The listing builds one solid part. Answer for the finished solid, in the listing's coordinates (mm). Face numbers are marked on the shaded views. A direction names the side the tool comes from. Coordinates: 2 decimals unless noted, no trailing zeros. Order: outer loops, then holes, each group sorted by start corner. A loop starts at its lowest first (then second) coordinate and runs counter-clockwise, first axis right, second up. Notation, with made-up numbers: (89.25, -25) -> (138.25, -25) arc R32 cw to (138.25, 2) -> close; hole circle Ø2 at (43, 5.5). An arc over 180 degrees is marked (long way). Write item = value, one per line.
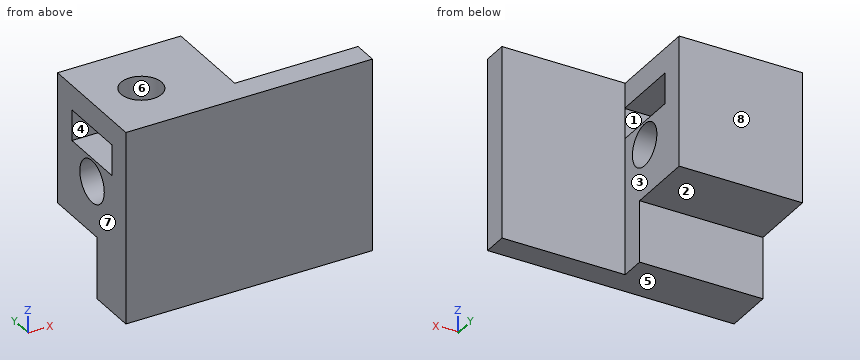
from build123d import *

# Parameters (mm, degrees)
RESSALTO_EXTRUS_O1_DEPTH             = 52.5
ESBO_O3_W                            = 10
ESBO_O3_H                            = 4
RESSALTO_EXTRUS_O2_DEPTH             = 5
ESBO_O4_R                            = 1.7
ESBO_O4_W                            = 2.5
ESBO_O4_H                            = 5.6
RESSALTO_EXTRUS_O3_DEPTH             = 10
ESBO_O5_R                            = 1.65
CORTE_EXTRUS_O1_DEPTH                = 6
RESSALTO_EXTRUS_O4_REACH             = 12.6
ESBO_O6_W                            = 10
ESBO_O6_H                            = 2
RESSALTO_EXTRUS_O4_DIRECTION_2_REACH = 117.6
ESBO_O7_W                            = 20
ESBO_O7_H                            = 110.6
CORTE_EXTRUS_O2_DEPTH                = 6.5
CORTE_EXTRUS_O2_DEPTH_BACK           = 5


with BuildPart() as part:
    # Esboço1 → Ressalto-extrusão1 (new body, symmetric)
    with BuildSketch(Plane.XY):
        Polygon((0, 0), (0, 2), (5, 2), (5, 4), (10, 4), (10, 2), (20, 2), (20, 0), align=None)
    extrude(amount=RESSALTO_EXTRUS_O1_DEPTH, both=True)

    # Esboço3 → Ressalto-extrusão2 (add)
    with BuildSketch(Plane.XY.offset(52.5)):
        with Locations((5, 2)):
            Rectangle(ESBO_O3_W, ESBO_O3_H)
    extrude(amount=-RESSALTO_EXTRUS_O2_DEPTH)

    # Esboço4 → Ressalto-extrusão3 (add, through all)
    with BuildSketch(Plane(origin=(10, 0, 0), x_dir=(0, 0, -1), z_dir=(1, 0, 0))):
        Polygon((-52.5, 9.5), (-63.1, 9.5), (-63.1, 0), (-52.5, 0), (-52.5, 3.742943079), align=None)
        with Locations((-56.7, 4.7)):
            Circle(ESBO_O4_R, mode=Mode.SUBTRACT)
        with Locations((-59.85, 4.7)):
            Rectangle(ESBO_O4_W, ESBO_O4_H, mode=Mode.SUBTRACT)
    ressalto_extrus_o3 = extrude(amount=-RESSALTO_EXTRUS_O3_DEPTH)

    # Esboço5 → Corte-extrusão1 (cut)
    with BuildSketch(Plane.XY.offset(63.1)):
        with Locations((4, 4.7)):
            Circle(ESBO_O5_R)
    corte_extrus_o1 = extrude(amount=-CORTE_EXTRUS_O1_DEPTH, mode=Mode.SUBTRACT)

    # Espelhar1: Ressalto-extrusão3, Corte-extrusão1 across plane
    add(ressalto_extrus_o3.mirror(Plane.XY))
    add(corte_extrus_o1.mirror(Plane.XY), mode=Mode.SUBTRACT)

    # Ressalto-extrusão4: up to this face of the body (flat: up to its plane)
    ressalto_extrus_o4_end = Plane(part.part.faces().sort_by_distance((5, 9.362068858, 63.1))[0])
    # Esboço6 → Ressalto-extrusão4 (add, up to the picked face)
    with BuildSketch(Plane.XY.offset(52.5), mode=Mode.PRIVATE) as ressalto_extrus_o4_sk1:
        with Locations((15, 1)):
            Rectangle(ESBO_O6_W, ESBO_O6_H)
    ressalto_extrus_o4_tool1 = split(extrude(ressalto_extrus_o4_sk1.sketch, amount=RESSALTO_EXTRUS_O4_REACH, mode=Mode.PRIVATE), bisect_by=ressalto_extrus_o4_end, keep=Keep.BOTH, mode=Mode.PRIVATE)
    add(ressalto_extrus_o4_tool1.solids().sort_by_distance((15, 1, 52.5))[0])

    # Ressalto-extrusão4 direction 2: up to this face of the body (flat: up to its plane)
    ressalto_extrus_o4_direction_2_end = Plane(part.part.faces().sort_by_distance((5, 9.362068858, -63.1))[0])
    # Esboço6 → Ressalto-extrusão4 direction 2 (add, up to the picked face)
    with BuildSketch(Plane.XY.offset(52.5), mode=Mode.PRIVATE) as ressalto_extrus_o4_direction_2_sk1:
        with Locations((15, 1)):
            Rectangle(ESBO_O6_W, ESBO_O6_H)
    ressalto_extrus_o4_direction_2_tool1 = split(extrude(ressalto_extrus_o4_direction_2_sk1.sketch, amount=-RESSALTO_EXTRUS_O4_DIRECTION_2_REACH, mode=Mode.PRIVATE), bisect_by=ressalto_extrus_o4_direction_2_end, keep=Keep.BOTH, mode=Mode.PRIVATE)
    add(ressalto_extrus_o4_direction_2_tool1.solids().sort_by_distance((15, 1, 52.5))[0])

    # Esboço7 → Corte-extrusão2 (cut, two sides)
    with BuildSketch(Plane(origin=(0, 4, 0), x_dir=(1, 0, 0), z_dir=(0, 1, 0))) as corte_extrus_o2_sk:
        with Locations((10, 7.8)):
            Rectangle(ESBO_O7_W, ESBO_O7_H)
    extrude(amount=CORTE_EXTRUS_O2_DEPTH, mode=Mode.SUBTRACT)
    extrude(corte_extrus_o2_sk.sketch, amount=-CORTE_EXTRUS_O2_DEPTH_BACK, mode=Mode.SUBTRACT)


solid = part.part
Q1. Find the intervals of material crossed by line 1 along Y through (x, z) = (4, 58.1); line 2 along Y through (x, z) = (7.75, 59.75); line 3 along Z through (x, y) = (9.25, 8), in increasing order.
The answers:
line_1 = 0 to 3.05, 6.35 to 9.5
line_2 = 0 to 1.9, 7.5 to 9.5
line_3 = 52.5 to 63.1
Q2. Each of these flat-tipped pins is pushed along its axis until it touches: pin 1 Ø3 at (x, y) = (3, 6) entering from -Z; pin 2 Ø5 at (x, z) = (16.5, 58) entering from +Y; pin 3 Ø2.5 at (x, z) = (3, 49) entering from +Y. Where does it stop, or does it pass through?
The answers:
pin_1 = 52.5
pin_2 = 2
pin_3 = 4
Q3. Section D-D, the plane x = 4 is taken. Give the vertices of the cut face in (y, z).
The answers:
outline = (0, 47.5) -> (4, 47.5) -> (4, 52.5) -> (9.5, 52.5) -> (9.5, 63.1) -> (6.35, 63.1) -> (6.35, 61.1) -> (7.5, 61.1) -> (7.5, 58.6) -> (6.35, 58.6) -> (6.35, 57.11) arc R1.7 cw (long way) to (3.05, 57.11) -> (3.05, 58.6) -> (1.9, 58.6) -> (1.9, 61.1) -> (3.05, 61.1) -> (3.05, 63.1) -> (0, 63.1) -> close
Q4. Section B-B, the plane z = 60.75 is taken. Give the vertices of the cut face in (x, y), plus the area to 3 significant figures.
The answers:
outline = (0, 0) -> (20, 0) -> (20, 2) -> (10, 2) -> (10, 1.9) -> (0, 1.9) -> close; (0, 7.5) -> (10, 7.5) -> (10, 9.5) -> (0, 9.5) -> close
area = 59.0 mm2
Q5. A tool of negligible diameter and unlimited length cuts with its end or side. For the marked faces 1, 2, 3, 4 and 5, from which of +Z, -Z, +X, -X, +Y, -Y can it reach the whole face along a straight path? Write none if from no direction.
The answers:
face_1 = -X
face_2 = -Z, +X, -X, +Y
face_3 = +Z, -Z, +X, +Y
face_4 = +X, -X
face_5 = -Z, +X, -X, +Y, -Y
Q6. Section A-A, the plane y = 4.7 is taken. Give the vertices of the cut face in (x, z).
The answers:
outline = (0, 52.5) -> (10, 52.5) -> (10, 55) -> (0, 55) -> close; (0, 58.4) -> (2.35, 58.4) -> (2.35, 58.6) -> (0, 58.6) -> close; (0, 61.1) -> (2.35, 61.1) -> (2.35, 63.1) -> (0, 63.1) -> close; (5.65, 58.4) -> (10, 58.4) -> (10, 58.6) -> (5.65, 58.6) -> close; (5.65, 61.1) -> (10, 61.1) -> (10, 63.1) -> (5.65, 63.1) -> close
Q7. The mould has two halves that part along X. Classify the marked faces 6, 7 and 8: released by +X, released by -X, zero draft, split by the parting line, or undercut.
The answers:
face_6 = undercut
face_7 = released by -X
face_8 = zero draft
Q8. Section C-C, the plane y = 2.25 is taken. Give the vertices of the cut face in (x, z), plus the area to 3 significant figures.
The answers:
outline = (0, 47.5) -> (10, 47.5) -> (10, 58.6) -> (0, 58.6) -> close; (0, 61.1) -> (10, 61.1) -> (10, 63.1) -> (0, 63.1) -> close
area = 131 mm2
